Model file for the job. Use its own axes, mm. Give positions to 0.01 mm unless a question says otherwise; leave off trailing zeros. Write each loop counter-clockwise with the first axis right and the second up, starting at its lowest first coordinate (ties: lowest second). Pieces come first, ordered by that corner, then holes. Notation, with made-up numbers: (-16, 20) - (34, 20) arc R29 ccw to (34, 41) - close; hole circle Ø1 at (-17, 27.25). An arc over 180 degrees is marked (long way). One line per item, written item: value. Start each with the question number.
(1) Cut at D-D, the plane z = 71. List the corners of the cut face in (x, y).
(2) Drop flat-ended pins along their axis: P1, Ø4, axis at y = 1.5, z = 58, coming from the +X side; P2, Ø4, axis at x = 37.5, y = 6, coming from the +Z side; P3, Ø3, axis at x = -56.5, y = 5.5, coming from the -Z side. Give the stop position or say it passes through.
(3) Cut at B-B, the plane z = 0. List the corners of the cut face in (x, y), and give its area (3 significant figures).
(4) Cut at A-A, the plane x = 0. List the corners of the cut face in (y, z), and give its area (3 significant figures).
(5) Probe L1, parallel to Z at x = 18.5, y = 9.5; L2, parallel to Z at x = 57, y = 2; L3, parallel to X at y = 5.75, z = 17.5. List the from-to ranges inside material, lowest first.
(6) Cut at C-C, the plane y = 9.5. List the corners of the cut face in (x, z).
from build123d import *

# Parameters (mm, degrees)
SKETCH1_R           = 95
BOSS_EXTRUDE1_DEPTH = 12
SKETCH2_R           = 25
CUT_EXTRUDE1_DEPTH  = 135.88513632
SKETCH3_R           = 8.457473765
CUT_EXTRUDE2_DEPTH  = 11.748282
CIRPATTERN1_START   = 0.251717624
CIRPATTERN1_DEPTH   = 11.748282376


# Read off the part's stored shape, not the designer's step: CirPattern1
with BuildPart() as part:
    # Sketch1 → Boss-Extrude1 (new body)
    with BuildSketch(Plane(origin=(0, 0, 0), x_dir=(1, 0, 0), z_dir=(0, 1, 0))):
        with Locations(Location((0, 0, 0), (0, 0, 270))):
            Circle(SKETCH1_R)
    extrude(amount=BOSS_EXTRUDE1_DEPTH)

    # Sketch2 → Cut-Extrude1 (cut, through all)
    with BuildSketch(Plane(origin=(0, 0, 0), x_dir=(1, 0, 0), z_dir=(0, 1, 0))):
        with Locations(Location((0, 0, 0), (0, 0, 270))):
            Circle(SKETCH2_R)
    extrude(amount=CUT_EXTRUDE1_DEPTH, mode=Mode.SUBTRACT)

    # Sketch3 → Cut-Extrude2 (cut)
    with BuildSketch(Plane(origin=(0, 12, 0), x_dir=(1, 0, 0), z_dir=(0, 1, 0))):
        with Locations((-19.300211782, 0)):
            Circle(SKETCH3_R)
    extrude(amount=-CUT_EXTRUDE2_DEPTH, mode=Mode.SUBTRACT)

    # CirPattern1 outline → CirPattern1 (cut)
    with BuildSketch(Plane(origin=(0, 0, 0), x_dir=(1, 0, 0), z_dir=(0, 1, 0)).offset(CIRPATTERN1_START)):
        with BuildLine():
            ThreePointArc((-21.93983937, 11.985134477), (-17.67766953, 17.67766953), (-11.985134477, 21.93983937))
            ThreePointArc((-11.985134477, 21.93983937), (-19.62764768, 19.62764768), (-21.93983937, 11.985134477))
        make_face()
        with BuildLine():
            ThreePointArc((7.039039335, 23.988579058), (0, 27.757685546), (-7.039039335, 23.988579058))
            ThreePointArc((-7.039039335, 23.988579058), (0, 25), (7.039039335, 23.988579058))
        make_face()
        with BuildLine():
            ThreePointArc((-11.985134477, -21.93983937), (-17.67766953, -17.67766953), (-21.93983937, -11.985134477))
            ThreePointArc((-21.93983937, -11.985134477), (-19.62764768, -19.62764768), (-11.985134477, -21.93983937))
        make_face()
        with BuildLine():
            ThreePointArc((21.93983937, 11.985134477), (19.62764768, 19.62764768), (11.985134477, 21.93983937))
            ThreePointArc((11.985134477, 21.93983937), (17.67766953, 17.67766953), (21.93983937, 11.985134477))
        make_face()
        with BuildLine():
            ThreePointArc((7.039039335, -23.988579058), (0, -25), (-7.039039335, -23.988579058))
            ThreePointArc((-7.039039335, -23.988579058), (0, -27.757685546), (7.039039335, -23.988579058))
        make_face()
        with BuildLine():
            ThreePointArc((23.988579058, -7.039039335), (27.757685546, 0), (23.988579058, 7.039039335))
            ThreePointArc((23.988579058, 7.039039335), (25, 0), (23.988579058, -7.039039335))
        make_face()
        with BuildLine():
            ThreePointArc((21.93983937, -11.985134477), (17.67766953, -17.67766953), (11.985134477, -21.93983937))
            ThreePointArc((11.985134477, -21.93983937), (19.62764768, -19.62764768), (21.93983937, -11.985134477))
        make_face()
    extrude(amount=CIRPATTERN1_DEPTH, mode=Mode.SUBTRACT)


solid = part.part
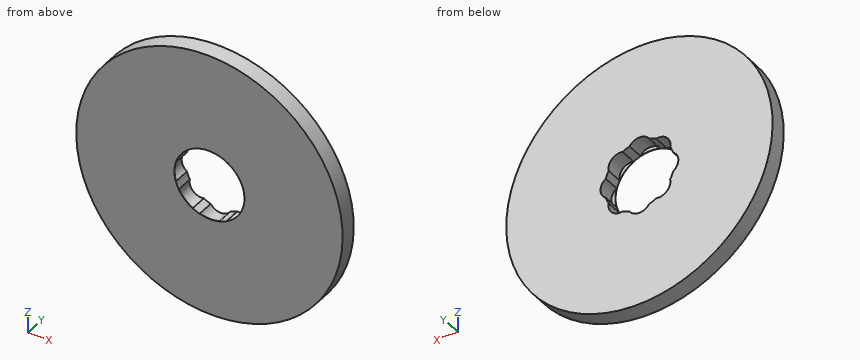
Answers follow:
1. outline: (-63.12, 0) - (63.12, 0) - (63.12, 12) - (-63.12, 12) - close
2. P1: stops at x = 76.74
2. P2: stops at z = 88.12
2. P3: stops at z = -77.46
3. outline: (-95, 0) - (-25, 0) - (-25, 0.25) - (-27.76, 0.25) - (-27.76, 12) - (-95, 12) - close; (25, 0) - (95, 0) - (95, 12) - (27.76, 12) - (27.76, 0.25) - (25, 0.25) - close
3. area: 1,620 mm²
4. outline: (0, -95) - (12, -95) - (12, -27.76) - (0.25, -27.76) - (0.25, -25) - (0, -25) - close; (0, 25) - (0.25, 25) - (0.25, 27.76) - (12, 27.76) - (12, 95) - (0, 95) - close
4. area: 1,620 mm²
5. L1: z = -93.18 to -20.57, 20.57 to 93.18
5. L2: z = -76 to 76
5. L3: x = -93.37 to -21.18, 21.18 to 93.37
6. outline: circle Ø190 at (0, 0); hole (-23.99, -7.04) arc R25 ccw to (-21.94, -11.99) arc R8.46 ccw to (-11.99, -21.94) arc R25 ccw to (-7.04, -23.99) arc R8.46 ccw to (7.04, -23.99) arc R25 ccw to (11.99, -21.94) arc R8.46 ccw to (21.94, -11.99) arc R25 ccw to (23.99, -7.04) arc R8.46 ccw to (23.99, 7.04) arc R25 ccw to (21.94, 11.99) arc R8.46 ccw to (11.99, 21.94) arc R25 ccw to (7.04, 23.99) arc R8.46 ccw to (-7.04, 23.99) arc R25 ccw to (-11.99, 21.94) arc R8.46 ccw to (-21.94, 11.99) arc R25 ccw to (-23.99, 7.04) arc R8.46 ccw to start
